from build123d import *

# Parameters (mm, degrees)
SKETCH_1_R          = 8
SKETCH_1_R_2        = 2.5
SKETCH_1_R_3        = 1.25
EXTRUDE_1_DEPTH     = 5
SKETCH_2_R          = 2.5
CUT_EXTRUDE_1_DEPTH = 2


with BuildPart() as part:
    # 草图1 → 凸台-拉伸1 (new body)
    with BuildSketch(Plane.XY):
        with Locations((-420.454135706, 61.666363326)):
            Circle(SKETCH_1_R)
        with Locations((-420.454135706, 61.666363326)):
            Circle(SKETCH_1_R_2, mode=Mode.SUBTRACT)
        with Locations((-420.454135706, 67.424629947)):
            Circle(SKETCH_1_R_3, mode=Mode.SUBTRACT)
        with Locations((-414.695869085, 61.666363326)):
            Circle(SKETCH_1_R_3, mode=Mode.SUBTRACT)
        with Locations((-420.454135706, 55.908096705)):
            Circle(SKETCH_1_R_3, mode=Mode.SUBTRACT)
        with Locations((-426.212402327, 61.666363326)):
            Circle(SKETCH_1_R_3, mode=Mode.SUBTRACT)
    extrude(amount=EXTRUDE_1_DEPTH)

    # 草图2 → 切除-拉伸1 (cut)
    with BuildSketch(Plane(origin=(0, 0, 0), x_dir=(-1, 0, 0), z_dir=(0, 0, -1))):
        with Locations((420.454135706, 67.424629947)):
            Circle(SKETCH_2_R)
        with Locations((426.212402327, 61.666363326)):
            Circle(SKETCH_2_R)
        with Locations((420.454135706, 55.908096705)):
            Circle(SKETCH_2_R)
        with Locations((414.695869085, 61.666363326)):
            Circle(SKETCH_2_R)
    extrude(amount=-CUT_EXTRUDE_1_DEPTH, mode=Mode.SUBTRACT)


solid = part.part
Geometry check sheet. Reference: the model listing, model coordinates, mm. A direction names the side the tool comes from. Round coordinates to 2 decimals unless told otherwise and drop trailing zeros. Order: outer loops, then holes, each group sorted by start corner. A loop starts at its lowest first (then second) coordinate and runs counter-clockwise, first axis right, second up. Notation, with made-up numbers: M 5.25,-34 L 12.25,-34 A21 cw 12.25,-24 Z; hole C -31,79 d10. An arc over 180 degrees is marked long. Answer in a Markdown table with one row per item. Add a question column.
Item 1: Sectioned sample at D-D, the plane z = 3.5. Enter the section's corners in (x, y).
Item 2: Set-up check for faces 5 (the face through (-419, 57, 2)), 6 (the face through (-422.95, 61.78, 2.46)): record each of +Z, -Z, +X, -X, +Y, -Y from which the full face is reachable in a straight line by a thin tool's end or side.
Item 3: Depth check by flat-ended pin: pin 1 Ø4 at (x, y) = (-414.7, 61.67) entering from -Z; pin 2 Ø2 at (x, y) = (-420.45, 55.91) entering from -Z; pin 3 Ø3 at (x, z) = (-425, 3) entering from +Y; pin 4 Ø1.5 at (y, z) = (59.5, 3.5) entering from +X. Enter the tip coordinate at first touch or a pass-through.
Item 4: Material ranges on L1, parallel to X at y = 61.75, z = 3.2; L2, parallel to Y at x = -420.75, z = 3.25; L3, parallel to Z at x = -426.5, y = 59.5, recorded low to high. Write a range as [from, to].
Item 5: Sectioned sample at B-B, the plane y = 66.5. Enter the section's corners in (x, z), plus the area to 3 significant figures.
Item 6: Sectioned sample at C-C, the plane z = 1.05. Enter the section's corners in (x, y).
Item 7: Draft check along X on faces 1 (the face through (-427, 63, 2)), 2 (the face through (-413.064, 58.602, 2.465)), 3 (the face through (-420.545, 58.406, 0.986)), 4 (the face through (-422, 64, 0)). Enter one of: released by +X, released by -X, zero draft, split by the parting line, or undercut.
Item 8: Sectioned sample at A-A, the plane x = -422. Enter the section's corners in (y, z), plus the area to 3 significant figures.
Filled in:
| question | item | result |
|---|---|---|
| 1 | outline | C -420.45,61.67 d16; hole C -426.21,61.67 d2.5; hole C -420.45,61.67 d5; hole C -420.45,55.91 d2.5; hole C -420.45,67.42 d2.5; hole C -414.7,61.67 d2.5 |
| 2 | face 5 | -Z |
| 2 | face 6 | +Z, -Z |
| 3 | pin 1 | stops at z = 2 |
| 3 | pin 2 | passes through |
| 3 | pin 3 | stops at y = 69.06 |
| 3 | pin 4 | stops at x = -412.58 |
| 4 | L1 | x = [-428.45, -427.46], [-424.97, -422.95], [-417.96, -415.94], [-413.45, -412.45] |
| 4 | L2 | y = [53.67, 54.69], [57.12, 59.18], [64.15, 66.21], [68.64, 69.66] |
| 4 | L3 | z = [2, 5] |
| 5 | outline | M -426.83,0 L -422.78,0 L -422.78,2 L -421.3,2 L -421.3,5 L -426.83,5 Z; M -419.61,2 L -418.13,2 L -418.13,0 L -414.08,0 L -414.08,5 L -419.61,5 Z |
| 5 | area | 49.4 mm² |
| 6 | outline | M -428.35,60.37 A8 ccw -421.75,53.77 A2.5 cw long -419.15,53.77 A8 ccw -412.56,60.37 A2.5 cw long -412.56,62.97 A8 ccw -419.15,69.56 A2.5 cw long -421.75,69.56 A8 ccw -428.35,62.97 A2.5 cw long Z; hole C -420.45,61.67 d5 |
| 7 | face 1 | undercut |
| 7 | face 2 | split by the parting line |
| 7 | face 3 | undercut |
| 7 | face 4 | zero draft |
| 8 | outline | M 53.82,0 L 53.94,0 L 53.94,2 L 57.87,2 L 57.87,0 L 59.7,0 L 59.7,5 L 53.82,5 Z; M 63.63,0 L 65.46,0 L 65.46,2 L 69.39,2 L 69.39,0 L 69.52,0 L 69.52,5 L 63.63,5 Z |
| 8 | area | 43.1 mm² |
